Here's how the part is built. I have some questions about the finished solid (model axes, mm). Face numbers are marked on the shaded views. A direction names the side the tool comes from. Give positions to 0.01 mm unless a question says otherwise; leave off trailing zeros. Order: outer loops, then holes, each group sorted by start corner. A loop starts at its lowest first (then second) coordinate and runs counter-clockwise, first axis right, second up. Notation, with made-up numbers: (6.5, 82.25) -> (35.5, 82.25) arc R16 cw to (35.5, 90.25) -> close; hole circle Ø6 at (77, 1.5). An arc over 180 degrees is marked (long way). Write each question's results on one line, items separated by ' | '. Start each with the question number.
Q1. Imagine slicing it at B-B, the plane y = 23.56. Please give me the cut outline in (x, z).
Q2. Imagine slicing it at A-A, the plane x = 26. Please give me the cut outline in (y, z) (3 decimals).
Q3. I'm going to push flat-ended pins straight in: pin 1 (22 mm diameter, centred on x = 14, y = 14, fed in from -Z); pin 2 (12 mm diameter, centred on y = 21, z = -13, fed in from -X); pin 3 (7.5 mm diameter, centred on x = 13, z = 5.5, fed in from -Y). Where does each tip first touch, or does it pass through?
Q4. Imagine slicing it at D-D, the plane z = -41. Please give me the cut outline in (x, y).
Q5. Thinking about a two-plate mould opening in Z: for the marked faces 1, 2 and 3, which applies, pulls with the +Z half, pulls with the -Z half, needs draft (parallel to the pull), parting line crosses it, or undercut?
Q6. I need wall thicknesses on line 1 along Y through (x, z) = (27, -15) (3 decimals); line 2 along Z through (x, y) = (27.5, 6.56); line 3 along Y through (x, z) = (28, -15) (3 decimals). Which ranges of each line are inside material? Lowest first, please. Write a range as [from, to].
Q7. Imagine slicing it at C-C, the plane z = -15. State how many separate pieces and enclosed holes the cut face has, then the cut area to 3 significant figures.
Q8. For the marked faces 4, 5, 6, 7 and 8, which set-ups out of +Z, -Z, +X, -X, +Y, -Y let a thin tool reach every point of the face, with its end or its side?
Autodesk Inventor part; units mm, degrees
ref_plane "Work Plane1" through (0, 0, -15) normal (0, 0, 1) x (1, 0, 0)
ref_plane "YZ Plane" through (0, 0, 0) normal (1, 0, 0) x (0, 1, 0)
ref_plane "XZ Plane" through (0, 0, 0) normal (0, 1, 0) x (-1, 0, 0)
sketch "Sketch1" plane through (0, 0, 0) normal (0, 0, 1) x (1, 0, 0)
  line L0 (0, 0) -> (25, 0)
  line L1 (25, 0) -> (25, 40)
  line L2 (25, 40) -> (0, 40)
  line L3 (0, 40) -> (0, 0)
  dimension "d1" = 25
  dimension "d2" = 40
  dimension "d3" = 25
extrude "Extrusion1" add sketch "Sketch1" against normal blind 30
sketch "Sketch2" plane through (25, 0, 0) normal (1, 0, 0) x (0, 0, -1)
  line L0 (0, 0) -> (30, 0)
  circle A0 centre (15, 6.56) radius 2.46
extrude "Extrusion2" cut sketch "Sketch2" against normal blind 30
sketch "Sketch3" plane through (0, 0, 0) normal (-1, 0, 0) x (0, 0, 1)
  line L0 (0, 0) -> (-30, 0)
  line L1 (-25.05, 0) -> (-4.95, 0)
  line L2 (-4.95, 0) -> (-4.95, 33.12)
  line L3 (-4.95, 33.12) -> (-25.05, 33.12)
  line L4 (-25.05, 33.12) -> (-25.05, 0)
  dimension "d11" = 20.1
extrude "Extrusion3" cut sketch "Sketch3" against normal blind 20
sketch "Sketch4" plane through (0, 0, 0) normal (0, -1, 0) x (1, 0, 0)
  line L0 (20, -4.95) -> (20, -25.05)
  line L1 (20, -15) -> (25, -15)
  line L2 (25, 0) -> (25, -30)
  line L3 (20, -8.025) -> (25, -8.025)
  line L4 (25, -8.025) -> (25, -21.975)
  line L5 (25, -21.975) -> (20, -21.975)
  line L6 (20, -21.975) -> (20, -8.025)
  line L7 (20, -8.025) -> (25, -21.975) construction
  line L8 (25, -8.025) -> (20, -21.975) construction
  line L9 (25, -12.54) -> (25, -17.46)
  point P0 (0, 0)
  point P1 (22.5, -15)
  dimension "d14" = 13.95
extrude "Extrusion4" add sketch "Sketch4" along normal blind 15
sketch "Sketch5" plane through (20, 0, 0) normal (-1, 0, 0) x (0, 0, 1)
  circle A0 centre (-15, 6.56) radius 2.46
  circle A1 centre (-15, 6.56) radius 4.7025
  circle A2 centre (-15, 6.56) radius 2.46
  circle A3 centre (-15, 6.56) radius 2.46
  point P0 (0, 0)
  dimension "d17" = 9.405
extrude "Extrusion5" cut sketch "Sketch5" against normal blind 2.1
sketch "Sketch6" plane through (25, 0, 0) normal (1, 0, 0) x (0, 0, -1)
  circle A0 centre (15, 6.56) radius 4.7025
  line L0 (15, 6.56) -> (15, 23.56)
  circle A1 centre (15, 23.56) radius 2.46
  point P0 (0, 0)
  dimension "d20" = 17
  dimension "d21" = 4.92
extrude "Extrusion6" cut sketch "Sketch6" against normal blind 10 contours A1
sketch "Sketch7" plane through (20, 0, 0) normal (-1, 0, 0) x (0, 0, 1)
  circle A0 centre (-15, 23.56) radius 2.46
  circle A1 centre (-15, 23.56) radius 4.7025
  point P0 (0, 0)
  dimension "d24" = 9.405
extrude "Extrusion7" cut sketch "Sketch7" against normal blind 2.1
sketch "Sketch9" plane through (25, 0, 0) normal (1, 0, 0) x (0, 0, -1)
  circle A0 centre (15, 6.56) radius 2.46
  circle A1 centre (15, 6.56) radius 2.46
  circle A2 centre (15, 23.56) radius 2.46
  circle A3 centre (15, 23.56) radius 2.46
  line L0 (30, 40) -> (30, 0)
  line L1 (30, 0) -> (30, 40)
  line L2 (30, 40) -> (0, 40)
  line L3 (0, 40) -> (0, 0)
  line L4 (0, 0) -> (8.025, 0)
  line L5 (21.975, 0) -> (21.975, -15)
  line L6 (21.975, -15) -> (8.025, -15)
  line L7 (8.025, -15) -> (8.025, 0)
  line L8 (0, 0) -> (8.025, 0)
  line L9 (21.975, 0) -> (30, 0)
extrude "Extrusion8" add sketch "Sketch9" along normal blind 5
sketch "Sketch10" plane through (0, 40, 0) normal (0, 1, 0) x (1, 0, 0)
  line L0 (0, 30) -> (30, 30)
  line L1 (30, 0) -> (0, 0)
  line L2 (0, 30) -> (30, 30)
  line L3 (30, 30) -> (30, 0)
  line L4 (30, 0) -> (0, 0)
  line L5 (0, 0) -> (0, 30)
extrude "Extrusion9" add sketch "Sketch10" along normal blind 30
sketch "Sketch12" plane through (30, 0, 0) normal (1, 0, 0) x (0, 0, -1)
  circle A0 centre (15, 6.56) radius 2.46
  line L0 (15, 6.56) -> (15, 15.06)
  circle A1 centre (15, 15.06) radius 2.525
  point P0 (0, 0)
  dimension "d31" = 8.5
  dimension "d33" = 5.05
extrude "Extrusion10" cut sketch "Sketch12" against normal blind 30 contours A1
sketch "Sketch14" plane through (0, 0, 0) normal (0, 0, 1) x (1, 0, 0)
  line L0 (30, 70) -> (0, 70)
  line L1 (0, 70) -> (0, 85)
  line L2 (-15, 100) -> (-23, 100)
  line L3 (30, 100) -> (15, 115)
  line L4 (-23, 115) -> (15, 115)
  line L5 (30, 0) -> (30, 70)
  line L6 (30, 100) -> (30, 70)
  line L7 (-20.5, 113.5) -> (-23, 115)
  line L8 (-20.5, 101.5) -> (-23, 100)
  line L9 (-18, 107.5) -> (-20.5, 101.5)
  line L10 (-18, 107.5) -> (-20.5, 113.5)
  arc A0 (0, 85) -> (-15, 100) centre (-15, 85) ccw
  point P0 (0, 0)
  point P1 (0, 100)
  dimension "d47" = 30
  dimension "d49" = 15
  dimension "d54" = 15
extrude "Extrusion12" add sketch "Sketch14" against normal blind 30
sketch "Sketch15" plane through (0, 0, -25.05) normal (-1, 0, 0) x (0, 0, 1)
  line L0 (0, 33.12) -> (20.1, 33.12)
  line L1 (20.1, 33.12) -> (20.1, 0)
  line L2 (0, 33.12) -> (20.1, 33.12)
  line L3 (20.1, 33.12) -> (20.1, 31.1)
  line L4 (20.1, 31.1) -> (0, 31.1)
  line L5 (0, 31.1) -> (0, 33.12)
  point P0 (25.05, 0)
  dimension "d57" = 2.02
extrude "Extrusion13" add sketch "Sketch15" against normal blind 20
sketch "Sketch17" plane through (0, 0, 0) normal (0, 0, 1) x (1, 0, 0)
  line L0 (-23, 115) -> (15, 115)
  line L1 (-23, 115) -> (15, 115)
  line L2 (30, 0) -> (30, 100)
  line L3 (15, 115) -> (30, 100)
  line L4 (30, 100) -> (30, 85)
  arc A0 (0, 85) -> (-15, 100) centre (-15, 85) ccw
  line L5 (30, 85) -> (0, 85)
  arc A1 (0, 85) -> (-15, 100) centre (-15, 85) ccw
  line L6 (-15, 100) -> (-23, 100)
  line L7 (-15, 100) -> (-23, 100)
  line L8 (-23, 100) -> (-20.5, 101.5)
  line L9 (-23, 100) -> (-20.5, 101.5)
  line L10 (-20.5, 101.5) -> (-18, 107.5)
  line L11 (-20.5, 101.5) -> (-18, 107.5)
  line L12 (-18, 107.5) -> (-20.5, 113.5)
  line L13 (-18, 107.5) -> (-20.5, 113.5)
  line L14 (-20.5, 113.5) -> (-23, 115)
  point P0 (0, 0)
extrude "Extrusion14" add sketch "Sketch17" along normal blind 15
ref_plane "Work Plane1" through (0, 0, -15) normal (0, 0, 1) x (1, 0, 0)
mirror "Mirror1" about plane through (0, 0, -15) normal (0, 0, 1) of "Extrusion14"
properties part number "12mm_x_60mm"
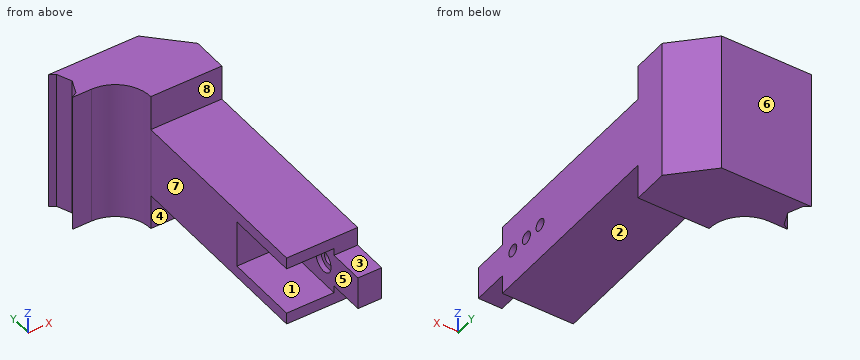
Geometry check:
1) outline: (0, -30) -> (30, -30) -> (30, -17.46) -> (22.1, -17.46) -> (22.1, -19.7) -> (20, -19.7) -> (20, -25.05) -> (0, -25.05) -> close; (0, -4.95) -> (20, -4.95) -> (20, -10.3) -> (22.1, -10.3) -> (22.1, -12.54) -> (30, -12.54) -> (30, 0) -> (0, 0) -> close
2) outline: (-15, -21.975) -> (0, -21.975) -> (0, -30) -> (85, -30) -> (85, -45) -> (104, -45) -> (104, 15) -> (85, 15) -> (85, 0) -> (0, 0) -> (0, -8.025) -> (-15, -8.025) -> close; hole circle Ø4.92 at (6.56, -15); hole circle Ø5.05 at (15.06, -15); hole circle Ø4.92 at (23.56, -15)
3) pin 1: z = -30 | pin 2: x = 20 | pin 3: y = 85
4) outline: (-23, 100) -> (-15, 100) arc R15 cw to (0, 85) -> (30, 85) -> (30, 100) -> (15, 115) -> (-23, 115) -> (-20.5, 113.5) -> (-18, 107.5) -> (-20.5, 101.5) -> close
5) face 1: undercut | face 2: pulls with the -Z half | face 3: pulls with the +Z half
6) line 1: [-15, 4.1], [9.02, 12.535], [17.585, 21.1], [26.02, 103] | line 2: [-30, -17.46], [-12.54, 0] | line 3: [-15, 4.1], [9.02, 12.535], [17.585, 21.1], [26.02, 102]
7) separate pieces: 4 | enclosed holes: 0 | area: 3,040 mm²
8) face 4: -Z, +X, -X, -Y | face 5: -X, -Y | face 6: +Z, -Z, +X, -X, +Y | face 7: +Z, -Z, -X, -Y | face 8: +Z, +X, -X, -Y
